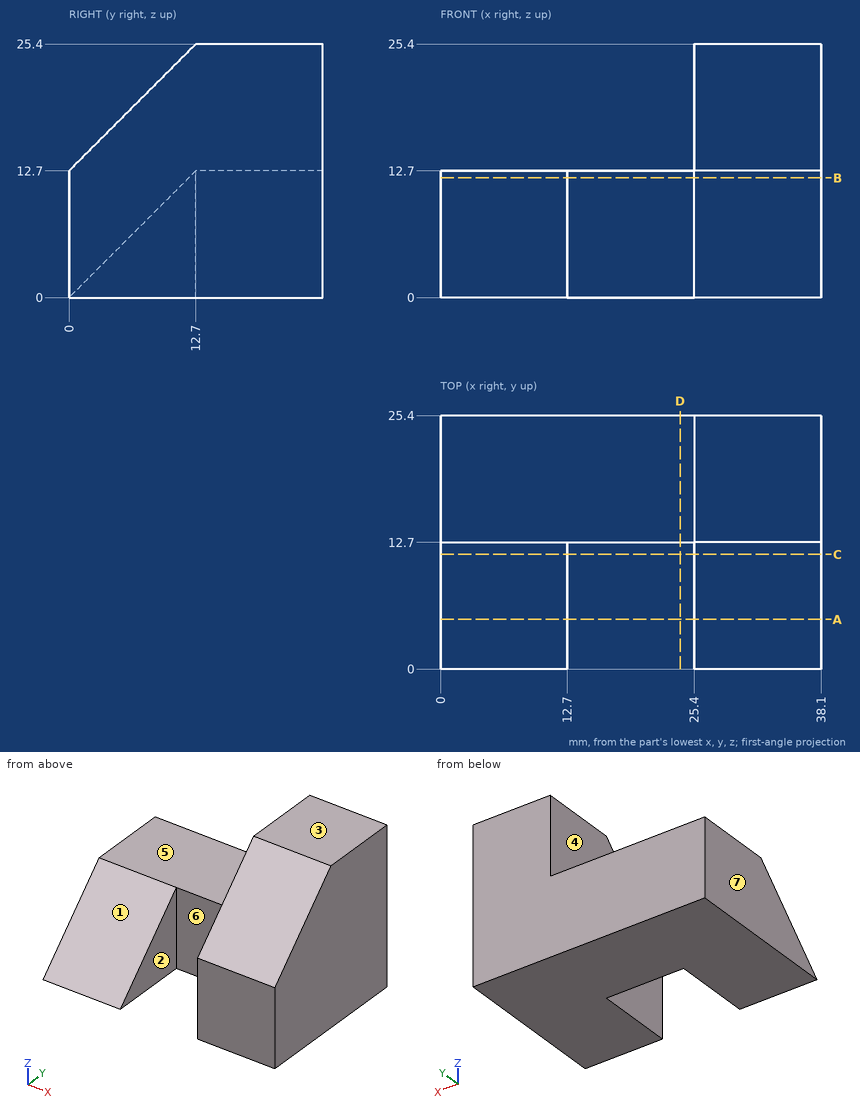
Source: three-view drawing plus pictorial views. Frame: mm from the lowest corner of the part. A direction names the side the tool comes from. Round coordinates to 2 decimals unless told otherwise and drop trailing zeros. Loops run counter-clockwise (first coordinate to the right, second up) from the corner with the lowest first, then second, coordinate; pieces in that order, holes last.
Q1. Access query for the marked faces 1, 2 and 3. Directions: +Z, -Z, +X, -X, +Y, -Y. A direction counts if a zero-diameter tool reaches every point of the face in a straight line with its end or side. Return the directions, or none.
Q2. First-contact query: P1, Ø6.5, axis at x = 16, y = 17, coming from the +Z side; P2, Ø2, axis at y = 18, z = 14.5, coming from the -X side; P3, Ø6, axis at x = 13, y = 5.5, coming from the -Z side; P4, Ø6.5, axis at x = 17.5, z = 4, coming from the -Y side. Flat tips, straight axial feed; report the tip coordinate or a pass-through.
Q3. Ray query, line 1 (Z direction, x = 21.5, y = 13.25); line 2 (X direction, y = 14, z = 22.25); line 3 (Y direction, x = 13, z = 6). Return the intervals inside material, ascending.
Q4. Section B-B, the plane z = 12. Return loops of the section in (x, y).
Q5. Section D-D, the plane x = 24. Return loops of the section in (y, z).
Q6. Section C-C, the plane y = 11.5. Return loops of the section in (x, z).
Q7. Section A-A, the plane y = 5. Return loops of the section in (x, z), plus the area to 3 significant figures.
Q8. Mould query, pull axis X, two halves, no side actions, for the marked faces 4, 5, 6 and 7. Classes: pulls with the +X half, pulls with the -X half, needs draft (parallel to the pull), parting line crosses it, or undercut.
Solutions:
1. face 1: +Z, -X, -Y
1. face 2: +Z, -Z, -Y
1. face 3: +Z, +X, -X, +Y, -Y
2. P1: stops at z = 12.7
2. P2: stops at x = 25.4
2. P3: stops at z = 0
2. P4: stops at y = 12.7
3. line 1: z = 0 to 12.7
3. line 2: x = 25.4 to 38.1
3. line 3: y = 12.7 to 25.4
4. outline: (0, 12) - (12.7, 12) - (12.7, 12.7) - (25.4, 12.7) - (25.4, 0) - (38.1, 0) - (38.1, 25.4) - (0, 25.4) - close
5. outline: (12.7, 0) - (25.4, 0) - (25.4, 12.7) - (12.7, 12.7) - close
6. outline: (0, 0) - (12.7, 0) - (12.7, 11.5) - (0, 11.5) - close; (25.4, 0) - (38.1, 0) - (38.1, 24.2) - (25.4, 24.2) - close
7. outline: (0, 0) - (12.7, 0) - (12.7, 5) - (0, 5) - close; (25.4, 0) - (38.1, 0) - (38.1, 17.7) - (25.4, 17.7) - close
7. area: 288 mm2
8. face 4: undercut
8. face 5: needs draft
8. face 6: undercut
8. face 7: pulls with the -X half
